from build123d import *

# Parameters (mm, degrees)
BOSS_EXTRUDE1_DEPTH      = 5
BOSS_EXTRUDE1_DEPTH_BACK = 5
SKETCH3_R                = 2.25
SKETCH3_R_2              = 1.35
CHAMFER1_SIZE            = 0.09
CHAMFER2_SIZE            = 0.135


with BuildPart() as part:
    # Sketch3 → Boss-Extrude1 (new, two sides: drawn at the far end of the back side and taken through both)
    with BuildSketch(Plane.XY.offset(-BOSS_EXTRUDE1_DEPTH_BACK)):
        Circle(SKETCH3_R)
        Circle(SKETCH3_R_2, mode=Mode.SUBTRACT)
    extrude(amount=BOSS_EXTRUDE1_DEPTH + BOSS_EXTRUDE1_DEPTH_BACK)

    # Chamfer1
    chamfer1_edges = [part.edges().sort_by_distance(p)[0] for p in [
        (-2.25, 0, -5),
        (-2.25, 0, 5),
    ]]
    chamfer(chamfer1_edges, length=CHAMFER1_SIZE)

    # Chamfer2
    chamfer2_edges = [part.edges().sort_by_distance(p)[0] for p in [
        (-1.35, 0, -5),
        (-1.35, 0, 5),
    ]]
    chamfer(chamfer2_edges, length=CHAMFER2_SIZE)


solid = part.part
Geometry: final body of the model. Coordinates: model frame, mm. Give positions to 0.01 mm unless a question says otherwise; leave off trailing zeros. Write each loop counter-clockwise with the first axis right and the second up, starting at its lowest first coordinate (ties: lowest second). Pieces come first, ordered by that corner, then holes. Notation, with made-up numbers: (7, -20) - (46, -20) arc R18 ccw to (46, -15) - close; hole circle Ø10 at (-16.75, 40). An arc over 180 degrees is marked (long way). Return JSON: item names as keys, results as strings. Group by question number.
1) Section C-C on z = 1. Return the cut outline in (x, y), plus the area to 3 significant figures.
2) First-contact query: P1, Ø1, axis at x = 1, z = 2.5, coming from the +Y side; P2, Ø2.5, axis at x = 0, y = 0, coming from the -Z side. Flat tips, straight axial feed; report the tip coordinate or a pass-through.
3) Line query: line 1 (Y direction, x = 0, z = 1.5); line 2 (Y direction, x = 1.8, z = 0); line 3 (Y direction, x = -1.2, z = 1.25). Output: solid intervals per line, ascending.
4) Section A-A on y = 0. Return the cut outline in (x, z) (3 decimals), plus the area to 3 significant figures.
5) Mould query, pull axis Y, two halves, no side actions, for faces 1 (the cylindrical face through (-0.29, 2.23, -0.07)), 2 (the cylindrical face through (-0.29, -1.32, -0.07)). Classes: released by +Y, released by -Y, zero draft, split by the parting line, or undercut.
Filled in:
{
 "1": {"outline": "circle Ø4.5 at (0, 0); hole circle Ø2.7 at (0, 0)", "area": "10.2 mm^2"},
 "2": {"P1": "stops at y = 2.19", "P2": "passes through"},
 "3": {"line 1": "y = -2.25 to -1.35, 1.35 to 2.25", "line 2": "y = -1.35 to 1.35", "line 3": "y = -1.9 to -0.62, 0.62 to 1.9"},
 "4": {"outline": "(-2.25, -4.91) - (-2.16, -5) - (-1.485, -5) - (-1.35, -4.865) - (-1.35, 4.865) - (-1.485, 5) - (-2.16, 5) - (-2.25, 4.91) - close; (1.35, -4.865) - (1.485, -5) - (2.16, -5) - (2.25, -4.91) - (2.25, 4.91) - (2.16, 5) - (1.485, 5) - (1.35, 4.865) - close", "area": "17.9 mm^2"},
 "5": {"face 1": "split by the parting line", "face 2": "undercut"}
}
